Geometry: final body of the model. Coordinates: model frame, mm. A direction names the side the tool comes from. Give positions to 0.01 mm unless a question says otherwise; leave off trailing zeros. Write each loop counter-clockwise with the first axis right and the second up, starting at its lowest first coordinate (ties: lowest second). Pieces come first, ordered by that corner, then holes.
Q1. Section B-B (y = -2.25). Return the cut outline in (x, z).
Q2. Line query: line 1 (Z direction, x = 2, y = 3.25); line 2 (Y direction, x = 9, z = 2). Output: solid intervals per line, ascending.
Q3. Section C-C (x = 10). Return the cut outline in (y, z), plus the area to 3 significant figures.
Q4. Section A-A (z = 0). Return the cut outline in (x, y), plus the area to 3 significant figures.
Q5. Section D-D (z = -2.25). Return the cut outline in (x, y), plus the area to 3 significant figures.
Q6. Reachability of faces 1 (the flat face through (1.7, 7, 14)), 2 (the flat face through (0, 4.3, 14)), 3 (the flat face through (0, -2, 10.75)), 4 (the flat face through (0, 0, -3.2)) from +Z, -Z, +X, -X, +Y, -Y: full face, straight path, thin tool, end or side. Return the list, or none.
Q7. Pin query (flat end, axial travel): pin 1 Ø3 at (y, z) = (-0.5, 12) entering from +X; pin 2 Ø1.6 at (y, z) = (7, 14.5) entering from +X; pin 3 Ø5 at (x, y) = (8.5, 5.5) entering from +Z. Return the tip coordinate at first contact, or that it passes through.
Q8. Mould query, pull axis Z, two halves, no side actions, for faces 5 (the flat face through (0, 2, 2.191)), 6 (the flat face through (-6, 1, -4.3)), 7 (the flat face through (4.35, 3, 7)). Classes: +Z half, -Z half, draft (parallel to the pull), parting line (faces both ways), or undercut.
from build123d import *

# Parameters (mm, degrees)
SKETCH2_W           = 8.6
SKETCH2_H           = 8.6
SKETCH2_W_2         = 6.4
SKETCH2_H_2         = 6.4
EXTRUDE_THIN1_DEPTH = 12.25
CHAMFER1_SIZE       = 0.3
BOSS_EXTRUDE1_START = -12.25
SKETCH3_W           = 0.6
SKETCH3_H           = 2.2
BOSS_EXTRUDE1_DEPTH = 5
SKETCH4_W           = 8.7
SKETCH4_H           = 1.8
BOSS_EXTRUDE2_DEPTH = 19.5
CUT_EXTRUDE1_REACH  = 25.32
SKETCH5_W           = 1.5
SKETCH5_H           = 1.8
CHAMFER2_SIZE       = 0.7
CHAMFER2_SIZE_2     = 1.923234194
SKETCH6_W           = 3.4
SKETCH6_H           = 1.5
BOSS_EXTRUDE3_DEPTH = 2
BOSS_EXTRUDE4_DEPTH = 8.7
CUT_EXTRUDE2_REACH  = 25.756
FILLET1_R           = 0.5
SKETCH8_W           = 4
SKETCH8_H           = 4.4
SKETCH8_W_2         = 2.6
SKETCH8_H_2         = 3
SKETCH8_W_3         = 8.4
SKETCH8_H_3         = 0.5
CUT_EXTRUDE3_DEPTH  = 0.3


with BuildPart() as part:
    # Sketch2 → Extrude-Thin1 (new, symmetric)
    with BuildSketch(Plane(origin=(0, 0, 0), x_dir=(0, 0, -1), z_dir=(1, 0, 0))):
        Rectangle(SKETCH2_W, SKETCH2_H)
        Rectangle(SKETCH2_W_2, SKETCH2_H_2, mode=Mode.SUBTRACT)
    extrude(amount=EXTRUDE_THIN1_DEPTH, both=True)

    # Chamfer1
    chamfer1_edges = [part.edges().sort_by_distance(p)[0] for p in [
        (-12.25, 0, -3.2),
        (0, -3.2, -3.2),
        (-12.25, 3.2, 0),
        (0, 3.2, -3.2),
        (-12.25, 0, 3.2),
        (0, 3.2, 3.2),
        (-12.25, -3.2, 0),
        (0, -3.2, 3.2),
        (12.25, 0, -3.2),
        (12.25, 3.2, 0),
        (12.25, 0, 3.2),
        (12.25, -3.2, 0),
    ]]
    chamfer(chamfer1_edges, length=CHAMFER1_SIZE)

    # Sketch3 → Boss-Extrude1 (add, symmetric)
    with BuildSketch(Plane(origin=(12.25, 0, 0), x_dir=(0, 0, -1), z_dir=(1, 0, 0)).offset(BOSS_EXTRUDE1_START)):
        with Locations((-1.891287847, 2.1)):
            Rectangle(SKETCH3_W, SKETCH3_H)
        with Locations((-1.891287847, -2.1)):
            Rectangle(SKETCH3_W, SKETCH3_H)
    extrude(amount=BOSS_EXTRUDE1_DEPTH, both=True)

    # Sketch4 → Boss-Extrude2 (add)
    with BuildSketch(Plane(origin=(0, 0, -4.3), x_dir=(-1, 0, 0), z_dir=(0, 0, -1))):
        with Locations((0, 5.2)):
            Rectangle(SKETCH4_W, SKETCH4_H)
    extrude(amount=-BOSS_EXTRUDE2_DEPTH)

    # Sketch5 → Cut-Extrude1 (cut, up to next)
    with BuildSketch(Plane(origin=(4.35, 0, 0), x_dir=(0, 0, -1), z_dir=(1, 0, 0)), mode=Mode.PRIVATE) as cut_extrude1_sk1:
        with Locations((1.95, 5.2)):
            Rectangle(SKETCH5_W, SKETCH5_H)
    cut_extrude1_tool1 = extrude(cut_extrude1_sk1.sketch, amount=-CUT_EXTRUDE1_REACH, mode=Mode.PRIVATE) & part.part
    add(cut_extrude1_tool1.solids().sort_by_distance((4.35, 5.2, -1.95))[0], mode=Mode.SUBTRACT)

    # Chamfer2
    # the kernel refuses this chamfer: 1.923234194, 0.7 mm, written as the material it takes off along each edge
    with BuildSketch(Plane(origin=(9.339244015, 6.1, -2.7), x_dir=(0, 0.09904090225205073, -0.9950833631817486), z_dir=(-1, 0, 0))) as chamfer2_piece_1_section:
        Polygon((CHAMFER2_SIZE * 0.995083363182, CHAMFER2_SIZE * 0.0990409022521), (-CHAMFER2_SIZE_2 * 0.0990409022324, CHAMFER2_SIZE_2 * 0.995083362984), (0, 0), align=None)
    chamfer2_piece_1 = extrude(amount=18.678488029, mode=Mode.PRIVATE)
    chamfer2_piece_1 = split(chamfer2_piece_1, bisect_by=Plane(origin=(0, 4.3, -2.919451718), z_dir=(0, 1, 0)), keep=Keep.TOP, mode=Mode.PRIVATE)
    add(chamfer2_piece_1, mode=Mode.SUBTRACT)

    # Sketch6 → Boss-Extrude3 (add)
    with BuildSketch(Plane.XY.offset(15.2)):
        with Locations((0, 6.85)):
            Rectangle(SKETCH6_W, SKETCH6_H)
    extrude(amount=-BOSS_EXTRUDE3_DEPTH)

    # Sketch7 → Boss-Extrude4 (add)
    with BuildSketch(Plane(origin=(4.35, 0, 0), x_dir=(0, 0, -1), z_dir=(1, 0, 0))):
        with BuildLine():
            ThreePointArc((-9.9, 3.7), (-9.862781283, 4.008842082), (-9.753256259, 4.3))
            Line((-9.753256259, 4.3), (-12.9, 4.3))
            Line((-12.9, 4.3), (-12.9, -4.3))
            Line((-12.9, -4.3), (-10.75, -4.3))
            Line((-10.75, -4.3), (-10.75, -0.56653645))
            ThreePointArc((-10.75, -0.56653645), (-10.913726036, 1.137708265), (-9.9, 2.5174241))
            Line((-9.9, 2.5174241), (-9.9, 3.7))
        make_face()
        with BuildLine():
            Line((-4.3, -4.3), (-4.3, 4.3))
            Line((-4.3, 4.3), (-7.446743741, 4.3))
            ThreePointArc((-7.446743741, 4.3), (-7.337218717, 4.008842082), (-7.3, 3.7))
            Line((-7.3, 3.7), (-7.3, 2.5174241))
            ThreePointArc((-7.3, 2.5174241), (-6.492869249, 1.648912529), (-6.2, 0.5))
            ThreePointArc((-6.2, 0.5), (-6.263335711, -0.047722558), (-6.45, -0.56653645))
            Line((-6.45, -0.56653645), (-6.45, -4.3))
            Line((-6.45, -4.3), (-4.3, -4.3))
        make_face()
    extrude(amount=-BOSS_EXTRUDE4_DEPTH)

    # Sketch7<3> → Cut-Extrude2 (cut, up to next)
    with BuildSketch(Plane(origin=(4.35, 0, 0), x_dir=(0, 0, -1), z_dir=(1, 0, 0)), mode=Mode.PRIVATE) as cut_extrude2_sk1:
        with BuildLine():
            Line((-9.753256259, 4.3), (-7.446743741, 4.3))
            ThreePointArc((-7.446743741, 4.3), (-8.6, 5), (-9.753256259, 4.3))
        make_face()
    cut_extrude2_tool1 = extrude(cut_extrude2_sk1.sketch, amount=-CUT_EXTRUDE2_REACH, mode=Mode.PRIVATE) & part.part
    add(cut_extrude2_tool1.solids().sort_by_distance((4.35, 4.587672, 8.6))[0], mode=Mode.SUBTRACT)

    # Fillet1
    fillet1_edges = [part.edges().sort_by_distance(p)[0] for p in [
        (0, -4.3, 10.75),
        (0, -4.3, 6.45),
    ]]
    fillet(fillet1_edges, radius=FILLET1_R)

    # Sketch8 → Cut-Extrude3 (cut)
    # profile 1 of 4: a face of its own
    with BuildSketch(Plane(origin=(0, 0, -4.3), x_dir=(-1, 0, 0), z_dir=(0, 0, -1))):
        with Locations((-6.2, 1.1)):
            Rectangle(SKETCH8_W, SKETCH8_H)
        with Locations((-6.2, 1.1)):
            Rectangle(SKETCH8_W_2, SKETCH8_H_2, mode=Mode.SUBTRACT)
    # profile 2 of 4: a face of its own
    with BuildSketch(Plane(origin=(0, 0, -4.3), x_dir=(-1, 0, 0), z_dir=(0, 0, -1))):
        with Locations((0, 2.05)):
            Rectangle(SKETCH8_W_3, SKETCH8_H_3)
    # profile 3 of 4: a face of its own
    with BuildSketch(Plane(origin=(0, 0, -4.3), x_dir=(-1, 0, 0), z_dir=(0, 0, -1))):
        with Locations((0, 0.15)):
            Rectangle(SKETCH8_W_3, SKETCH8_H_3)
    # profile 4 of 4: a face of its own
    with BuildSketch(Plane(origin=(0, 0, -4.3), x_dir=(-1, 0, 0), z_dir=(0, 0, -1))):
        with Locations((6.2, 1.1)):
            Rectangle(SKETCH8_W, SKETCH8_H)
        with Locations((6.2, 1.1)):
            Rectangle(SKETCH8_W_2, SKETCH8_H_2, mode=Mode.SUBTRACT)
    extrude(amount=-CUT_EXTRUDE3_DEPTH, mode=Mode.SUBTRACT)


solid = part.part
Computed:
1. outline: (-12.25, -4.3) - (12.25, -4.3) - (12.25, -3.5) - (11.95, -3.2) - (-11.95, -3.2) - (-12.25, -3.5) - close; (-12.25, 3.5) - (-11.95, 3.2) - (11.95, 3.2) - (12.25, 3.5) - (12.25, 4.3) - (4.35, 4.3) - (4.35, 6.45) - (-4.35, 6.45) - (-4.35, 4.3) - (-12.25, 4.3) - close; (-5, 1.59) - (5, 1.59) - (5, 2.19) - (-5, 2.19) - close; (-4.35, 10.75) - (4.35, 10.75) - (4.35, 12.9) - (-4.35, 12.9) - close
2. line 1: z = -4.3 to 7.3, 9.9 to 12.9
2. line 2: y = -4.3 to -3.2, 3.2 to 4.3
3. outline: (-4.3, -4.3) - (4.3, -4.3) - (4.3, 4.3) - (-4.3, 4.3) - close; hole (-3.2, -2.9) - (-2.9, -3.2) - (2.9, -3.2) - (3.2, -2.9) - (3.2, 2.9) - (2.9, 3.2) - (-2.9, 3.2) - (-3.2, 2.9) - close
3. area: 33.2 mm2
4. outline: (-12.25, -4.3) - (12.25, -4.3) - (12.25, -3.5) - (11.95, -3.2) - (-11.95, -3.2) - (-12.25, -3.5) - close; (-12.25, 3.5) - (-11.95, 3.2) - (11.95, 3.2) - (12.25, 3.5) - (12.25, 4.3) - (4.35, 4.3) - (4.35, 6.1) - (-4.35, 6.1) - (-4.35, 4.3) - (-12.25, 4.3) - close
4. area: 69.4 mm2
5. outline: (-12.25, -4.3) - (12.25, -4.3) - (12.25, -3.5) - (11.95, -3.2) - (-11.95, -3.2) - (-12.25, -3.5) - close; (-12.25, 3.5) - (-11.95, 3.2) - (11.95, 3.2) - (12.25, 3.5) - (12.25, 4.3) - (-12.25, 4.3) - close
5. area: 53.7 mm2
6. face 1: +Z, -Z, +X, +Y
6. face 2: +Z, +X, -X, -Y
6. face 3: +X, -X, -Y
6. face 4: +X, -X
7. pin 1: stops at x = 4.35
7. pin 2: stops at x = 1.7
7. pin 3: stops at z = 4.3
8. face 5: undercut
8. face 6: -Z half
8. face 7: draft
